The model under review builds one solid part; all positions refer to its coordinate system, in mm. Face numbers are marked on the shaded views. A direction names the side the tool comes from. Coordinates: 2 decimals unless noted, no trailing zeros. Write each loop counter-clockwise with the first axis right and the second up, starting at its lowest first coordinate (ties: lowest second). Pieces come first, ordered by that corner, then holes. Notation, with made-up numbers: (56, 69.5) - (79, 69.5) arc R17 cw to (79, 101.5) - close; hole circle Ø3 at (27, -10.5). An arc over 180 degrees is marked (long way). Put each result on its own line as item: value.
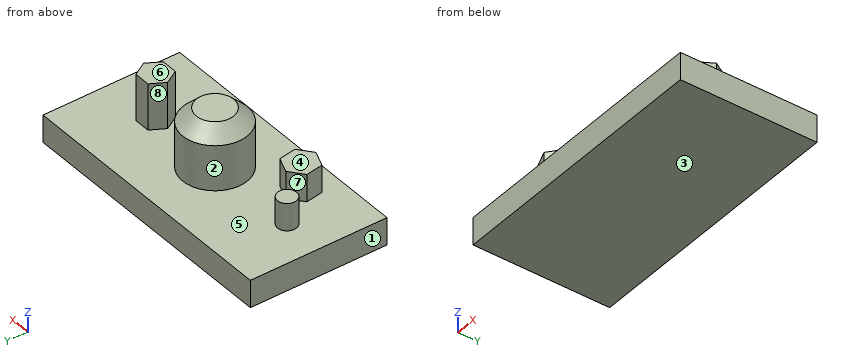
from build123d import *

# Parameters (mm, degrees)
F0_R      = 30
F1_DEPTH  = 80
F2_W      = 254
F2_H      = 127
F3_DEPTH  = 25.4
F4_SIZE   = 12.7
F5_R      = 8.764352
F6_DEPTH  = 25.4
F8_DEPTH  = 42.926
F10_DEPTH = 25.4


with BuildPart() as f1:
    # F0 (on Top) → F1 (new body)
    with BuildSketch(Plane.XY):
        Circle(F0_R)
    extrude(amount=F1_DEPTH)

    # F2 (on Top) → F3 (join)
    with BuildSketch(Plane.XY):
        Rectangle(F2_W, F2_H)
    extrude(amount=F3_DEPTH)

    # F4
    f4_edges = [f1.edges().sort_by_distance(p)[0] for p in [
        (-30, 0, 80),
    ]]
    chamfer(f4_edges, length=F4_SIZE)

    # F5 (on face) → F6 (join)
    with BuildSketch(Plane.XY.offset(25.4)):
        with Locations((-88.250794, 0)):
            Circle(F5_R)
    extrude(amount=F6_DEPTH)

    # F7 (on face) → F8 (join)
    with BuildSketch(Plane.XY.offset(25.4)):
        Polygon((80.111949, 12.750117), (65.389382, 12.750117), (58.028098, 0), (65.389382, -12.750117), (80.111949, -12.750117), (87.473232, 0), align=None)
    extrude(amount=F8_DEPTH)

    # F9 (on face) → F10 (join)
    with BuildSketch(Plane.XY.offset(25.4)):
        Polygon((-48.244875, -23.636972), (-63.256118, -17.863414), (-75.761787, -27.976753), (-73.256213, -43.863649), (-58.24497, -49.637207), (-45.739301, -39.523868), align=None)
    extrude(amount=F10_DEPTH)


solid = f1.part
1. To check wall thickness, follow probe 1 along Z at (x, y) = (78, 8.5); probe 2 along Z at (x, y) = (60, 21); probe 3 along X at (y, z) = (-0.5, 57). State the ranges of each line that lie inside material, in increasing order.
Determined:
probe 1: z = 0 to 68.33
probe 2: z = 0 to 25.4
probe 3: x = -30 to 30, 58.32 to 87.18
2. Consider section D-D on y = 44.5. State the section outline as (x, z) points.
Determined:
outline: (-127, 0) - (127, 0) - (127, 25.4) - (-127, 25.4) - close
3. Machinability: for the marked faces 4, 5, 6, 7 and 8, which of the approach directions +Z, -Z, +X, -X, +Y, -Y give a long, thin tool a straight path to every point of the face, cutting with its end or side? Answer none if there is none.
Determined:
face 4: +Z, -X, +Y, -Y
face 5: +Z
face 6: +Z, +X, +Y, -Y
face 7: +Z, -X, +Y
face 8: +Z, +Y
4. Consider section B-B on y = -35.5. State the section outline as (x, z) points, plus the area to 3 significant figures.
Determined:
outline: (-127, 0) - (127, 0) - (127, 25.4) - (-46.37, 25.4) - (-46.37, 50.8) - (-74.58, 50.8) - (-74.58, 25.4) - (-127, 25.4) - close
area: 7,170 mm^2
5. Consider section A-A on x = 0. State the section outline as (y, z) points, plus the area to 3 significant figures.
Determined:
outline: (-63.5, 0) - (63.5, 0) - (63.5, 25.4) - (30, 25.4) - (30, 67.3) - (17.3, 80) - (-17.3, 80) - (-30, 67.3) - (-30, 25.4) - (-63.5, 25.4) - close
area: 6,340 mm^2
6. Consider section C-C on x = -91.5. State the section outline as (y, z) points, plus the area to 3 significant figures.
Determined:
outline: (-63.5, 0) - (63.5, 0) - (63.5, 25.4) - (8.14, 25.4) - (8.14, 50.8) - (-8.14, 50.8) - (-8.14, 25.4) - (-63.5, 25.4) - close
area: 3,640 mm^2
7. For pin 1 Ø7.5 at (x, z) = (73.5, 50.5) entering from +Y; pin 2 Ø13 at (x, y) = (74.5, -1) entering from +Z; pin 3 Ø12 at (x, z) = (74.5, 56.5) entering from -Y, all flat-tipped, find the tip position at first contact; note any pin that passes through.
Determined:
pin 1: stops at y = 12.75
pin 2: stops at z = 68.33
pin 3: stops at y = -12.75
8. The part is to be moulded in two halves that separate along X. For the marked faces 1, 2 and 3, say which applies: +X half, -X half, draft (parallel to the pull), parting line (faces both ways), or undercut.
Determined:
face 1: -X half
face 2: undercut
face 3: draft
